CAD build for the part. Positions are in the model's coordinates, mm. Coordinates: 2 decimals unless noted, no trailing zeros. Order: outer loops, then holes, each group sorted by start corner. A loop starts at its lowest first (then second) coordinate and runs counter-clockwise, first axis right, second up. Notation, with made-up numbers: (-7.75, 73) - (5.25, 73) arc R16 cw to (5.25, 88) - close; hole circle Ø9 at (11, 79.25). An arc over 180 degrees is marked (long way). Use one line per item in the form item = value.
```python
from build123d import *

# Parameters (mm, degrees)
SKETCH1_R                      = 76
SKETCH1_R_2                    = 65
BOSS_EXTRUDE1_DEPTH            = 1.6
F_8_0_199_DIAMETER_HOLE1_D     = 5.0546
F_8_0_199_DIAMETER_HOLE1_DEPTH = 8.481444958
F_8_0_199_DIAMETER_HOLE1_TIP   = 1.518555042


with BuildPart() as part:
    # Sketch1 → Boss-Extrude1 (new body)
    with BuildSketch(Plane.XY):
        Circle(SKETCH1_R)
        Circle(SKETCH1_R_2, mode=Mode.SUBTRACT)
    extrude(amount=BOSS_EXTRUDE1_DEPTH)

    # #8 (0.199) Diameter Hole1
    with Locations(Plane(origin=(-27.318507381, 65.952711024, 1.6), x_dir=(1, 0, 0), z_dir=(0, 0, 1))):
        with Locations((0, 0), (54.637014762, 0), (93.271218405, -38.634203643), (93.271218405, -93.271218405), (54.637014762, -131.905422048), (0, -131.905422048), (-38.634203643, -93.271218405), (-38.634203643, -38.634203643)):
            Hole(F_8_0_199_DIAMETER_HOLE1_D / 2, depth=F_8_0_199_DIAMETER_HOLE1_DEPTH)
            with Locations((0, 0, -(F_8_0_199_DIAMETER_HOLE1_DEPTH + F_8_0_199_DIAMETER_HOLE1_TIP / 2))):  # 118° drill point
                Cone(0, F_8_0_199_DIAMETER_HOLE1_D / 2, F_8_0_199_DIAMETER_HOLE1_TIP, mode=Mode.SUBTRACT)


solid = part.part
```
Item 1: Two-plate mould, pull along X, no slides. Class faces 1 (the face through (-63.428, -27.207, 0.789)), 2 (the face through (35.069, -67.425, 0.789)), 3 (the face through (22, -62, 1.6)): +X half, -X half, draft (parallel to the pull), parting line (faces both ways), or undercut.
Derived:
face_1 = undercut
face_2 = parting line
face_3 = draft
Item 2: Cut at C-C, the plane z = 0.65. State how many separate pieces and enclosed holes the cut face has, plus the area to 3 significant figures.
Derived:
separate_pieces = 1
enclosed_holes = 9
area = 4,710 mm²
Item 3: Cut at A-A, the plane x = 0. Write the cut outline in (y, z), plus the area to 3 significant figures.
Derived:
outline = (-76, 0) - (-65, 0) - (-65, 1.6) - (-76, 1.6) - close; (65, 0) - (76, 0) - (76, 1.6) - (65, 1.6) - close
area = 35.2 mm²
Item 4: Drill centre lines: line 1 (X direction, y = 27.5, z = 1); line 2 (X direction, y = -7, z = 0.95); line 3 (Y direction, x = -29, z = 0.6). Where is each one in solid material? Low to high. Write a range as [from, to].
Derived:
line_1 = [-70.85, -68.47], [-63.43, -58.9], [58.9, 63.43], [68.47, 70.85]
line_2 = [-75.68, -64.62], [64.62, 75.68]
line_3 = [-70.25, -67.84], [-64.07, -58.17], [58.17, 64.07], [67.84, 70.25]
